from build123d import *

# Parameters (mm, degrees)
SKETCH1_W           = 45.72
SKETCH1_H           = 58.42
BOSS_EXTRUDE1_DEPTH = 6.35
SKETCH2_R           = 1.905
CUT_EXTRUDE1_DEPTH  = 40.859352933
SKETCH3_W           = 36.327462092
SKETCH3_H           = 46.418423785
BOSS_EXTRUDE2_DEPTH = 5.08
SKETCH4_R           = 7.62
SKETCH4_R_2         = 5.08
BOSS_EXTRUDE3_DEPTH = 12.7
FILLET1_R           = 2.54
SKETCH5_R           = 10.795
CUT_EXTRUDE2_DEPTH  = 8.89
SKETCH6_R           = 1.016
CUT_EXTRUDE3_DEPTH  = 19.05
CUT_EXTRUDE4_START  = -19.05
SKETCH4_2_R         = 5.08
CUT_EXTRUDE4_DEPTH  = 19.05


with BuildPart() as part:
    # Sketch1 → Boss-Extrude1 (new body)
    with BuildSketch(Plane(origin=(0, 0, 0), x_dir=(1, 0, 0), z_dir=(0, 1, 0))):
        with Locations((2.874210526, -0.559043062)):
            Rectangle(SKETCH1_W, SKETCH1_H)
    extrude(amount=BOSS_EXTRUDE1_DEPTH)

    # Sketch2 → Cut-Extrude1 (cut, through all)
    with BuildSketch(Plane(origin=(0, 6.35, 0), x_dir=(1, 0, 0), z_dir=(0, 1, 0))):
        with Locations(Location((-8.555789474, 14.045956938, 0), (0, 0, 270))):
            Circle(SKETCH2_R)
        with Locations(Location((14.304210526, 14.045956938, 0), (0, 0, 270))):
            Circle(SKETCH2_R)
        with Locations(Location((-8.555789474, -15.164043062, 0), (0, 0, 270))):
            Circle(SKETCH2_R)
        with Locations(Location((14.304210526, -15.164043062, 0), (0, 0, 270))):
            Circle(SKETCH2_R)
    extrude(amount=-CUT_EXTRUDE1_DEPTH, mode=Mode.SUBTRACT)

    # Sketch3 → Boss-Extrude2 (add)
    with BuildSketch(Plane.XZ):
        with Locations((2.874210526, 0.559043062)):
            Rectangle(SKETCH3_W, SKETCH3_H)
    extrude(amount=BOSS_EXTRUDE2_DEPTH)

    # Sketch4 → Boss-Extrude3 (add)
    with BuildSketch(Plane.XZ.offset(5.08)):
        with Locations(Location((2.874210526, 0.559043062, 0), (0, 0, 270))):
            Circle(SKETCH4_R)
        with Locations(Location((2.874210526, 0.559043062, 0), (0, 0, 270))):
            Circle(SKETCH4_R_2, mode=Mode.SUBTRACT)
    extrude(amount=BOSS_EXTRUDE3_DEPTH)

    # Fillet1
    fillet1_edges = [part.edges().sort_by_distance(p)[0] for p in [
        (-19.985789474, 3.175, -28.650956938),
        (25.734210526, 3.175, -28.650956938),
        (25.734210526, 3.175, 29.769043062),
        (-19.985789474, 3.175, 29.769043062),
    ]]
    fillet(fillet1_edges, radius=FILLET1_R)

    # Sketch5 → Cut-Extrude2 (cut)
    with BuildSketch(Plane(origin=(0, 6.35, 0), x_dir=(1, 0, 0), z_dir=(0, 1, 0))):
        with Locations(Location((2.874210526, -0.559043062, 0), (0, 0, 270))):
            Circle(SKETCH5_R)
    extrude(amount=-CUT_EXTRUDE2_DEPTH, mode=Mode.SUBTRACT)

    # Sketch6 → Cut-Extrude3 (cut)
    with BuildSketch(Plane(origin=(0, 6.35, 0), x_dir=(1, 0, 0), z_dir=(0, 1, 0))):
        with Locations(Location((-13.290250492, -0.559043062, 0), (0, 0, 270))):
            Circle(SKETCH6_R)
        with Locations(Location((2.874210526, 15.605417956, 0), (0, 0, 270))):
            Circle(SKETCH6_R)
        with Locations(Location((19.038671544, -0.559043062, 0), (0, 0, 270))):
            Circle(SKETCH6_R)
        with Locations(Location((2.874210526, -16.72350408, 0), (0, 0, 270))):
            Circle(SKETCH6_R)
    extrude(amount=-CUT_EXTRUDE3_DEPTH, mode=Mode.SUBTRACT)

    # Sketch4_2 → Cut-Extrude4 (cut)
    with BuildSketch(Plane.XZ.offset(5.08).offset(CUT_EXTRUDE4_START)):
        with Locations(Location((2.874210526, 0.559043062, 0), (0, 0, 90))):
            Circle(SKETCH4_2_R)
    extrude(amount=CUT_EXTRUDE4_DEPTH, mode=Mode.SUBTRACT)


solid = part.part
Geometry: final body of the model. Coordinates: model frame, mm. A direction names the side the tool comes from. Round coordinates to 2 decimals unless told otherwise and drop trailing zeros. Loops run counter-clockwise (first coordinate to the right, second up) from the corner with the lowest first, then second, coordinate; pieces in that order, holes last.
Q1. Section B-B on x = 9.5. Return loops of the section in (y, z).
Q2. Section A-A on z = 22. Return loops of the section in (x, y).
Q3. Access query for faces 1 (the flat face through (21.038, -3, 0)), 2 (the flat face through (3, -3, -22.65)), 3 (the flat face through (-9, 0, -14)). Directions: +Z, -Z, +X, -X, +Y, -Y. A direction counts if a zero-diameter tool reaches every point of the face in a straight line with its end or side. Return the directions, or none.
Q4. Section D-D on y = -11. Return loops of the section in (x, z).
Q5. Section C-C on y = 3.75. State how many separate pieces and enclosed holes the cut face has, plus the area to 3 significant figures.
Q6. Pull-direction query (X, two-part tool) for faces 4 (the flat face through (25.734, 3, 1)), 5 (the flat face through (-18, 0, 0)), 6 (the flat face through (14, 0, 15)), 7 (the cylindrical face through (-1.76, -11.34, 6.61)); classes: released by +X, released by -X, zero draft, split by the parting line, or undercut.
Q7. Material intervals for L1, parallel to X at y = -7, z = 0.5; L2, parallel to Z at x = 14, y = 2.25; L3, parallel to Y at x = -17.5, z = -6, sorted ascending.
Q8. Pin query (flat end, axial travel): P1, Ø1.6, axis at x = -13.29, z = 0.56, coming from the +Y side; P2, Ø13, axis at x = 2.87, z = 0.56, coming from the +Y side; P3, Ø3, axis at x = -8.56, z = -14.05, coming from the +Y side; P4, Ø3, axis at x = -2.5, y = -3, coming from the -Z side. Return the tip coordinate at first contact, or that it passes through.
Evaluation:
1. outline: (-17.78, -3.2) - (-5.08, -3.2) - (-5.08, -22.65) - (0, -22.65) - (0, -28.65) - (6.35, -28.65) - (6.35, -7.96) - (-2.54, -7.96) - (-2.54, 9.08) - (6.35, 9.08) - (6.35, 29.77) - (0, 29.77) - (0, 23.77) - (-5.08, 23.77) - (-5.08, 4.32) - (-17.78, 4.32) - close
2. outline: (-19.99, 0) - (-15.29, 0) - (-15.29, -5.08) - (21.04, -5.08) - (21.04, 0) - (25.73, 0) - (25.73, 6.35) - (-19.99, 6.35) - close
3. face 1: +Z, -Z, +X, -Y
3. face 2: -Z, +X, -X, -Y
3. face 3: +Y
4. outline: circle Ø15.24 at (2.87, 0.56); hole circle Ø10.16 at (2.87, 0.56)
5. separate pieces: 1
5. enclosed holes: 9
5. area: 2,240 mm2
6. face 4: released by +X
6. face 5: zero draft
6. face 6: undercut
6. face 7: split by the parting line
7. L1: x = -4.75 to -2.21, 7.95 to 10.49
7. L2: z = -28.65 to -15.93, -12.17 to 13.28, 17.04 to 29.77
7. L3: y = 0 to 6.35
8. P1: passes through
8. P2: stops at y = -2.54
8. P3: stops at y = 0
8. P4: stops at z = -22.65
